For this review, take the finished solid that the model builds, in its own axes (mm). Face numbers are marked on the shaded views. A direction names the side the tool comes from. Give positions to 0.01 mm unless a question says otherwise; leave off trailing zeros. Loops run counter-clockwise (first coordinate to the right, second up) from the corner with the lowest first, then second, coordinate; pieces in that order, holes last. Notation, with made-up numbers: (60.25, -17.5) -> (67.25, -17.5) arc R22 cw to (67.25, -5.5) -> close; hole circle Ø5 at (0.25, 73). An arc over 180 degrees is marked (long way). One line per question, with ' | ' between items. Start each with the question number.
(1) Consider section C-C (y = 2.2). Write out the cut boundary in (x, z), and give its area (3 significant figures).
(2) Consider section D-D (x = 21). Write out the cut boundary in (y, z), and give its area (3 significant figures).
(3) Wall thickness on probe 1 along Z at (x, y) = (15.7, 1.25); probe 2 along X at (y, z) = (2.2, 0); probe 3 along Z at (x, y) = (20, 1): over which ranges is each line inside the solid? List them lowest first.
(4) Consider section A-A (z = -5). Write out the cut boundary in (x, y), and give its area (3 significant figures).
(5) Consider section B-B (x = 15.7). Write out the cut boundary in (y, z), and give its area (3 significant figures).
(6) Draft analysis for pull direction X (two halves, no side actions). For the marked faces 3, 4 and 5, state which applies: +X half, -X half, draft (parallel to the pull), parting line (faces both ways), or undercut.
(7) Tool access review of the marked faces 1 and 2: name each direction out of +Z, -Z, +X, -X, +Y, -Y from which nothing blocks a thin tool from reaching the whole face with its end or side.
(8) Insertion check: P1, Ø0.9, axis at x = 3, y = 1, coming from the -Z side; P2, Ø3.5, axis at x = 15.7, z = -10, coming from the +Y side. Each pin has a flat end and moves straight along its axis. Give the tip position at first contact, or say it passes through.
from build123d import *

# Parameters (mm, degrees)
ESBO_O1_W                  = 40
ESBO_O1_H                  = 25
RESSALTO_EXTRUS_O1_DEPTH   = 3
ESBO_O7_W                  = 3
ESBO_O7_H                  = 8
CORTE_EXTRUS_O3_DEPTH      = 43.014878317
PERFIL_CORTE_W             = 23
PERFIL_CORTE_H             = 12.4
CORTE_PRINCIPAL_DEPTH      = 76.288119648
FURO_DE_DI_METRO_3_0_3_1_D = 3
ESBO_O6_W                  = 3
ESBO_O6_H                  = 5
CORTE_EXTRUS_O2_DEPTH      = 92.50164688
FILETE1_R                  = 4


with BuildPart() as part:
    # Esboço1 → Ressalto-extrusão1 (new body)
    with BuildSketch(Plane(origin=(0, 0, 0), x_dir=(1, 0, 0), z_dir=(0, 1, 0))):
        with Locations((20, 0)):
            Rectangle(ESBO_O1_W, ESBO_O1_H)
    extrude(amount=RESSALTO_EXTRUS_O1_DEPTH)

    # Esboço7 → Corte-extrusão3 (cut, through all)
    with BuildSketch(Plane(origin=(0, 0, 0), x_dir=(1, 0, 0), z_dir=(0, 1, 0))):
        with Locations((36, 0)):
            Rectangle(ESBO_O7_W, ESBO_O7_H)
    extrude(amount=CORTE_EXTRUS_O3_DEPTH, mode=Mode.SUBTRACT)

    # Perfil Corte → Corte Principal (cut, through all)
    with BuildSketch(Plane(origin=(62.223874948, 0, 29.778722149), x_dir=(-1, 0, 0), z_dir=(0, -1, 0))):
        with Locations((46.523874948, 29.778722149)):
            Rectangle(PERFIL_CORTE_W, PERFIL_CORTE_H)
    extrude(amount=-CORTE_PRINCIPAL_DEPTH, mode=Mode.SUBTRACT)

    # Furo de diâmetro Ø3.0 (3)1 (through all)
    with Locations(Plane(origin=(84.444031263, 0, 22.610638925), x_dir=(-1, 0, 0), z_dir=(0, -1, 0))):
        with Locations((68.744031263, 32.610638925), (68.744031263, 12.610638925)):
            Hole(FURO_DE_DI_METRO_3_0_3_1_D / 2)

    # Esboço6 → Corte-extrusão2 (cut, through all)
    with BuildSketch(Plane(origin=(84.444031263, 0, 22.610638925), x_dir=(-1, 0, 0), z_dir=(0, -1, 0))):
        with Locations((81.744031263, 22.610638925)):
            Rectangle(ESBO_O6_W, ESBO_O6_H)
    extrude(amount=-CORTE_EXTRUS_O2_DEPTH, mode=Mode.SUBTRACT)

    # Filete1
    filete1_edges = [part.edges().sort_by_distance(p)[0] for p in [
        (0, 1.5, -12.5),
        (40, 1.5, -12.5),
        (40, 1.5, 12.5),
        (0, 1.5, 12.5),
    ]]
    fillet(filete1_edges, radius=FILETE1_R)


solid = part.part
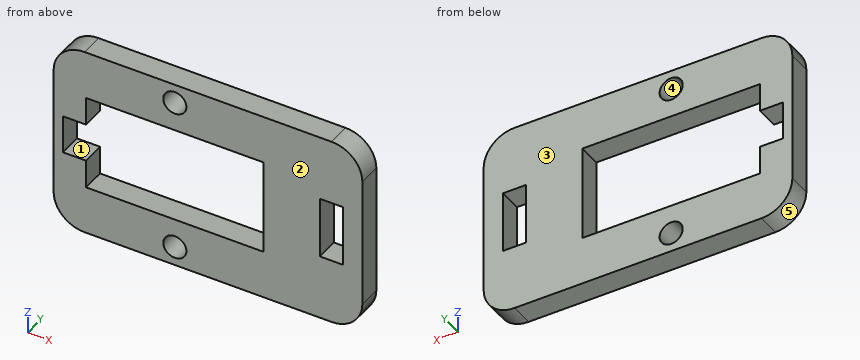
A:
1) outline: (0, -8.5) arc R4 ccw to (4, -12.5) -> (36, -12.5) arc R4 ccw to (40, -8.5) -> (40, 8.5) arc R4 ccw to (36, 12.5) -> (4, 12.5) arc R4 ccw to (0, 8.5) -> close; hole (1.2, -2.5) -> (4.2, -2.5) -> (4.2, -6.2) -> (27.2, -6.2) -> (27.2, 6.2) -> (4.2, 6.2) -> (4.2, 2.5) -> (1.2, 2.5) -> close; hole circle Ø3 at (15.7, -10); hole circle Ø3 at (15.7, 10); hole (34.5, -4) -> (37.5, -4) -> (37.5, 4) -> (34.5, 4) -> close | area: 648 mm^2
2) outline: (0, -12.5) -> (3, -12.5) -> (3, -6.2) -> (0, -6.2) -> close; (0, 6.2) -> (3, 6.2) -> (3, 12.5) -> (0, 12.5) -> close | area: 37.8 mm^2
3) probe 1: z = -12.5 to -11.5, -8.5 to -6.2, 6.2 to 8.5, 11.5 to 12.5 | probe 2: x = 0 to 1.2, 27.2 to 34.5, 37.5 to 40 | probe 3: z = -12.5 to -6.2, 6.2 to 12.5
4) outline: (0, 0) -> (4.2, 0) -> (4.2, 3) -> (0, 3) -> close; (27.2, 0) -> (40, 0) -> (40, 3) -> (27.2, 3) -> close | area: 51.0 mm^2
5) outline: (0, -12.5) -> (3, -12.5) -> (3, -11.5) -> (0, -11.5) -> close; (0, -8.5) -> (3, -8.5) -> (3, -6.2) -> (0, -6.2) -> close; (0, 6.2) -> (3, 6.2) -> (3, 8.5) -> (0, 8.5) -> close; (0, 11.5) -> (3, 11.5) -> (3, 12.5) -> (0, 12.5) -> close | area: 19.8 mm^2
6) face 3: draft | face 4: undercut | face 5: -X half
7) face 1: +Y, -Y | face 2: +Z, -Z, +X, -X, -Y
8) P1: stops at z = -12.46 | P2: stops at y = 3
